Geometry: final body of the model. Coordinates: model frame, mm. Round coordinates to 2 decimals unless told otherwise and drop trailing zeros. Write each loop counter-clockwise with the first axis right and the second up, starting at its lowest first coordinate (ties: lowest second). Pieces come first, ordered by that corner, then holes.
from build123d import *

# Parameters (mm, degrees)
F1_DEPTH      = 12.7
F2_R          = 5.08
F4_DEPTH      = 220.001
F4_DEPTH_BACK = 220.001


with BuildPart() as f1:
    # F0 (on Right) → F1 (new body, symmetric)
    with BuildSketch(Plane.YZ):
        with BuildLine():
            Line((-25.4, 220), (-31.75, 220))
            Line((-31.75, 220), (-31.75, -220))
            Line((-31.75, -220), (-25.4, -220))
            Line((-25.4, -220), (-19.05, -65.95))
            Line((-19.05, -65.95), (-19.05, -81.698))
            ThreePointArc((-19.05, -81.698), (-16.222995, -88.522995), (-9.398, -91.35))
            Line((-9.398, -91.35), (3.048, -91.35))
            ThreePointArc((3.048, -91.35), (5.382867, -90.382867), (6.35, -88.048))
            Line((6.35, -88.048), (6.35, -78.65))
            ThreePointArc((6.35, -78.65), (5.382867, -76.315133), (3.048, -75.348))
            Line((3.048, -75.348), (0, -75.348))
            Line((0, -75.348), (0, -85))
            Line((0, -85), (-6.35, -85))
            Line((-6.35, -85), (-6.35, 85))
            Line((-6.35, 85), (0, 85))
            Line((0, 85), (0, 75.348))
            Line((0, 75.348), (3.048, 75.348))
            ThreePointArc((3.048, 75.348), (5.382867, 76.315133), (6.35, 78.65))
            Line((6.35, 78.65), (6.35, 88.048))
            ThreePointArc((6.35, 88.048), (5.382867, 90.382867), (3.048, 91.35))
            Line((3.048, 91.35), (-9.398, 91.35))
            ThreePointArc((-9.398, 91.35), (-16.222995, 88.522995), (-19.05, 81.698))
            Line((-19.05, 81.698), (-19.05, 65.95))
            Line((-19.05, 65.95), (-25.4, 220))
        make_face()
    extrude(amount=F1_DEPTH, both=True)

    # F2
    f2_edges = [f1.edges().sort_by_distance(p)[0] for p in [
        (12.7, -31.75, 0),
        (-12.7, -31.75, 0),
    ]]
    fillet(f2_edges, radius=F2_R)

    # F3 (on Top) → F4 (cut, two sides)
    with BuildSketch(Plane.XY) as f4_sk:
        with BuildLine():
            Line((10.16, -26.67), (10.16, 6.35))
            Line((10.16, 6.35), (-10.16, 6.35))
            Line((-10.16, 6.35), (-10.16, -26.67))
            ThreePointArc((-10.16, -26.67), (-9.416051, -28.466051), (-7.62, -29.21))
            Line((-7.62, -29.21), (7.62, -29.21))
            ThreePointArc((7.62, -29.21), (9.416051, -28.466051), (10.16, -26.67))
        make_face()
    extrude(amount=F4_DEPTH, mode=Mode.SUBTRACT)
    extrude(f4_sk.sketch, amount=-F4_DEPTH_BACK, mode=Mode.SUBTRACT)


solid = f1.part
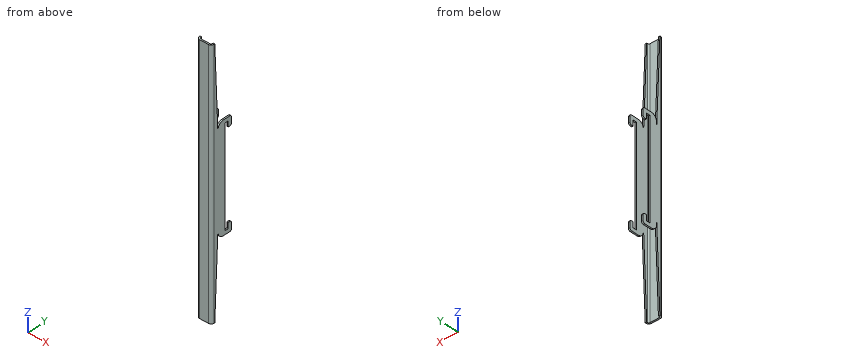
1) Section A-A on z = -36.5. Output: boundary loops of the cut face in (x, y).
2) Section B-B on x = -3.25. Output: boundary loops of the cut face in (y, z), plus the area to 3 significant figures.
3) Section C-C on z = -141.5. Output: boundary loops of the cut face in (x, y), plus the area to 3 significant figures.
4) Line query: probe 1 along X at (y, z) = (-14, 6); probe 2 along Y at (x, z) = (5.75, 59.5); probe 3 along X at (y, z) = (-28.5, 20.5). Output: solid intervals per line, ascending.
5) First-contact query: P1, Ø2, axis at x = -11, z = -81, coming from the -Y side; P2, Ø1.3, axis at x = -11, z = -74, coming from the -Y side; P3, Ø0.8, axis at x = 11.5, z = -73.5, coming from the -Y side. Flat tips, straight axial feed; report the tip coordinate or a pass-through.
Filled in:
1. outline: (-12.7, -26.67) arc R5.08 ccw to (-7.62, -31.75) - (7.62, -31.75) arc R5.08 ccw to (12.7, -26.67) - (12.7, -6.35) - (10.16, -6.35) - (10.16, -26.67) arc R2.54 cw to (7.62, -29.21) - (-7.62, -29.21) arc R2.54 cw to (-10.16, -26.67) - (-10.16, -6.35) - (-12.7, -6.35) - close
2. outline: (-31.75, -220) - (-29.21, -220) - (-29.21, 220) - (-31.75, 220) - close
2. area: 1,120 mm2
3. outline: (-12.7, -26.67) arc R5.08 ccw to (-7.62, -31.75) - (7.62, -31.75) arc R5.08 ccw to (12.7, -26.67) - (12.7, -22.16) - (10.16, -22.16) - (10.16, -26.67) arc R2.54 cw to (7.62, -29.21) - (-7.62, -29.21) arc R2.54 cw to (-10.16, -26.67) - (-10.16, -22.16) - (-12.7, -22.16) - close
3. area: 92.0 mm2
4. probe 1: x = -12.7 to -10.16, 10.16 to 12.7
4. probe 2: y = -31.75 to -29.21
4. probe 3: x = -12.36 to -9.38, 9.38 to 12.36
5. P1: stops at y = -31.16
5. P2: stops at y = -30.95
5. P3: stops at y = -30.37
